from build123d import *

# Parameters (mm, degrees)
BOSS_EXTRUDE1_DEPTH     = 10
SKETCH2_W               = 20
SKETCH2_H               = 2
CUT_EXTRUDE1_DEPTH      = 11
SKETCH3_R               = 1.5
CUT_EXTRUDE2_DEPTH      = 1
CUT_EXTRUDE2_DEPTH_BACK = 21.3


with BuildPart() as part:
    # Sketch1 → Boss-Extrude1 (new body)
    with BuildSketch(Plane.XY):
        Polygon((-4, 0), (4, 0), (10.5, 13), (18, 13), (18, 20.3), (-18, 20.3), (-18, 13), (-10.5, 13), align=None)
    extrude(amount=BOSS_EXTRUDE1_DEPTH)

    # Sketch2 → Cut-Extrude1 (cut, through all)
    with BuildSketch(Plane.XY.offset(10)):
        with Locations((0, 19.3)):
            Rectangle(SKETCH2_W, SKETCH2_H)
    extrude(amount=-CUT_EXTRUDE1_DEPTH, mode=Mode.SUBTRACT)

    # Sketch3 → Cut-Extrude2 (cut, two sides)
    with BuildSketch(Plane(origin=(0, 20.3, 0), x_dir=(1, 0, 0), z_dir=(0, 1, 0))) as cut_extrude2_sk:
        with Locations((-13.5, -5)):
            Circle(SKETCH3_R)
        with Locations((13.5, -5)):
            Circle(SKETCH3_R)
    extrude(amount=CUT_EXTRUDE2_DEPTH, mode=Mode.SUBTRACT)
    extrude(cut_extrude2_sk.sketch, amount=-CUT_EXTRUDE2_DEPTH_BACK, mode=Mode.SUBTRACT)


solid = part.part
Could you check a few things on this model? Use its own coordinates, in mm. A direction names the side the tool comes from. Coordinates: 2 decimals unless noted, no trailing zeros. Loops run counter-clockwise (first coordinate to the right, second up) from the corner with the lowest first, then second, coordinate; pieces in that order, holes last. Notation, with made-up numbers: (-37, 22) -> (17, 22) arc R19 cw to (17, 50) -> close; hole circle Ø5 at (57, 58). An arc over 180 degrees is marked (long way). Answer in a Markdown table with one row per item.
(1) For faces 1 (the face through (0, 18.3, 5)), 2 (the face through (-15, 20.3, 4)), 3 (the face through (-15, 13, 4)), 4 (the face through (15, 13, 4)), which set-ups out of +Z, -Z, +X, -X, +Y, -Y let a thin tool reach every point of the face, with its end or its side?
Results found:
| item | result |
|---|---|
| face 1 | +Z, -Z, +Y |
| face 2 | +Z, -Z, +X, -X, +Y |
| face 3 | +Z, -Z, -X, -Y |
| face 4 | +Z, -Z, +X, -Y |
(2) Imagine slicing it at B-B (x = 13.5). List the corners of the cut face in (y, z) for me, plus the area to 3 significant figures.
Results found:
| item | result |
|---|---|
| outline | (13, 0) -> (20.3, 0) -> (20.3, 3.5) -> (13, 3.5) -> close; (13, 6.5) -> (20.3, 6.5) -> (20.3, 10) -> (13, 10) -> close |
| area | 51.1 mm^2 |
(3) Imagine slicing it at D-D (z = 8). List the corners of the cut face in (x, y) for me.
Results found:
| item | result |
|---|---|
| outline | (-18, 13) -> (-10.5, 13) -> (-4, 0) -> (4, 0) -> (10.5, 13) -> (18, 13) -> (18, 20.3) -> (10, 20.3) -> (10, 18.3) -> (-10, 18.3) -> (-10, 20.3) -> (-18, 20.3) -> close |
(4) Thinking about a two-plate mould opening in Z: for faces 5 (the face through (-10, 19, 5)), 6 (the face through (12, 17, 5)), 7 (the face through (-15, 17, 5)), 8 (the face through (0, 13, 0)), which applies, released by +Z, released by -Z, zero draft, split by the parting line, or undercut?
Results found:
| item | result |
|---|---|
| face 5 | zero draft |
| face 6 | undercut |
| face 7 | undercut |
| face 8 | released by -Z |
(5) Imagine slicing it at A-A (y = 19.25). List the corners of the cut face in (x, z) for me.
Results found:
| item | result |
|---|---|
| outline | (-18, 0) -> (-10, 0) -> (-10, 10) -> (-18, 10) -> close; (10, 0) -> (18, 0) -> (18, 10) -> (10, 10) -> close; hole circle Ø3 at (-13.5, 5); hole circle Ø3 at (13.5, 5) |
(6) If I drill on probe 1 along X at (y, z) = (17.25, 5); probe 2 along X at (y, z) = (18.75, 5); probe 3 along Z at (x, y) = (-13.5, 18), over which ranges is the centre line in solid material (lowest first)?
Results found:
| item | result |
|---|---|
| probe 1 | x = -18 to -15, -12 to 12, 15 to 18 |
| probe 2 | x = -18 to -15, -12 to -10, 10 to 12, 15 to 18 |
| probe 3 | z = 0 to 3.5, 6.5 to 10 |
(7) Imagine slicing it at C-C (z = 5). List the corners of the cut face in (x, y) for me.
Results found:
| item | result |
|---|---|
| outline | (-18, 13) -> (-15, 13) -> (-15, 20.3) -> (-18, 20.3) -> close; (-12, 13) -> (-10.5, 13) -> (-4, 0) -> (4, 0) -> (10.5, 13) -> (12, 13) -> (12, 20.3) -> (10, 20.3) -> (10, 18.3) -> (-10, 18.3) -> (-10, 20.3) -> (-12, 20.3) -> close; (15, 13) -> (18, 13) -> (18, 20.3) -> (15, 20.3) -> close |
(8) Will these pins go through, and if not, where does the flat tip stop? pin 1 Ø2 at (x, z) = (13.5, 6) entering from -Y; pin 2 Ø6 at (x, z) = (2.5, 3) entering from +Y; pin 3 Ø6 at (x, z) = (-13, 3) entering from -Y.
Results found:
| item | result |
|---|---|
| pin 1 | stops at y = 13 |
| pin 2 | stops at y = 18.3 |
| pin 3 | stops at y = 12 |
